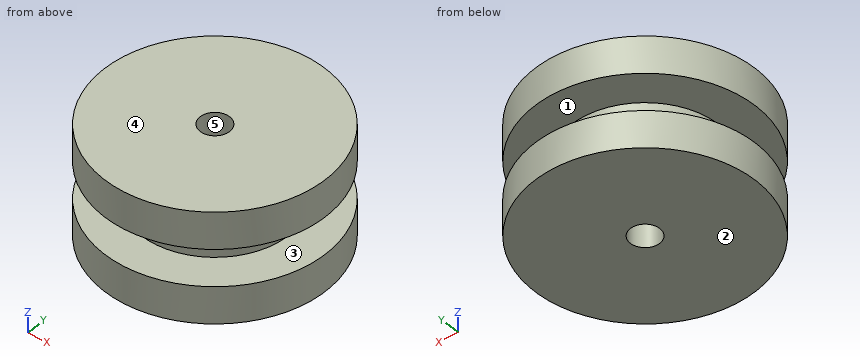
```python
from build123d import *

# Parameters (mm, degrees)
SKETCH1_R          = 20
EXTRUDE1_DEPTH     = 5
SKETCH2_R          = 30
EXTRUDE2_DEPTH     = 10
EXTRUDE3_START     = 10
SKETCH3_R          = 30
EXTRUDE3_DEPTH     = 10
SKETCH4_R          = 4
CUT_EXTRUDE1_DEPTH = 30


with BuildPart() as part:
    # Sketch1 → Extrude1 (new, symmetric)
    with BuildSketch(Plane.XY):
        Circle(SKETCH1_R)
    extrude(amount=EXTRUDE1_DEPTH, both=True)

    # Sketch2 → Extrude2 (add)
    with BuildSketch(Plane.XY.offset(5)):
        Circle(SKETCH2_R)
    extrude(amount=EXTRUDE2_DEPTH)

    # Sketch3 → Extrude3 (add)
    with BuildSketch(Plane(origin=(0, 0, -5), x_dir=(-1, 0, 0), z_dir=(0, 0, -1)).offset(EXTRUDE3_START)):
        with Locations(Location((0, 0, 0), (0, 0, 180))):
            Circle(SKETCH3_R)
    extrude(amount=-EXTRUDE3_DEPTH)

    # Sketch4 → Cut-Extrude1 (cut)
    with BuildSketch(Plane(origin=(0, 0, -15), x_dir=(-1, 0, 0), z_dir=(0, 0, -1))):
        Circle(SKETCH4_R)
    extrude(amount=-CUT_EXTRUDE1_DEPTH, mode=Mode.SUBTRACT)


solid = part.part
```
The listing builds one solid part. Answer for the finished solid, in the listing's coordinates (mm). Face numbers are marked on the shaded views. A direction names the side the tool comes from. Coordinates: 2 decimals unless noted, no trailing zeros. Write each loop counter-clockwise with the first axis right and the second up, starting at its lowest first coordinate (ties: lowest second). Pieces come first, ordered by that corner, then holes. Notation, with made-up numbers: (55.5, 24.5) - (73.5, 24.5) arc R26 cw to (73.5, 62.5) - close; hole circle Ø4 at (64, 45.25). An arc over 180 degrees is marked (long way). Return JSON: item names as keys, results as strings. Group by question number.
Q1. Flat-ended cylindrical pins translate along their axes: pin 1 Ø10 at (x, z) = (17.5, -9.5) entering from +Y; pin 2 Ø12 at (y, z) = (19, -4) entering from -X; pin 3 Ø8 at (x, z) = (-11, -12) entering from +Y. Find the tip coordinate at first contact, or state that the pin passes through.
Q2. The part is cut by section C-C on z = -3.75. Write down the section's boundary in (x, y), and give its area (3 significant figures).
Q3. For a pull along Z with two mould halves and no side action, classify the marked faces 3, 4 and 5 as +Z half, -Z half, draft (parallel to the pull), parting line (faces both ways), or undercut.
Q4. The part is cut by section D-D on x = 16. Write down the section's boundary in (y, z).
Q5. Find the intervals of material crossed by line 1 along Z through (x, y) = (24.5, 13); line 2 along Y through (x, z) = (0, -7.75); line 3 along Y through (x, z) = (0, 0.75), in increasing order. Write a range as [from, to].
Q6. The part is cut by section A-A on x = 0. Write down the section's boundary in (y, z).
Q7. Which of the six approach directions +Z, -Z, +X, -X, +Y, -Y give full straight-line access (tool end or side, diameter ignored) to the marked faces 1 and 2?
Evaluation:
{
 "1": {"pin 1": "stops at y = 27.27", "pin 2": "stops at x = -27", "pin 3": "stops at y = 29.17"},
 "2": {"outline": "circle Ø40 at (0, 0); hole circle Ø8 at (0, 0)", "area": "1,210 mm2"},
 "3": {"face 3": "undercut", "face 4": "+Z half", "face 5": "draft"},
 "4": {"outline": "(-25.38, -15) - (25.38, -15) - (25.38, -5) - (12, -5) - (12, 5) - (25.38, 5) - (25.38, 15) - (-25.38, 15) - (-25.38, 5) - (-12, 5) - (-12, -5) - (-25.38, -5) - close"},
 "5": {"line 1": "z = [-15, -5], [5, 15]", "line 2": "y = [-30, -4], [4, 30]", "line 3": "y = [-20, -4], [4, 20]"},
 "6": {"outline": "(-30, -15) - (-4, -15) - (-4, 15) - (-30, 15) - (-30, 5) - (-20, 5) - (-20, -5) - (-30, -5) - close; (4, -15) - (30, -15) - (30, -5) - (20, -5) - (20, 5) - (30, 5) - (30, 15) - (4, 15) - close"},
 "7": {"face 1": "none", "face 2": "-Z, +X, -X, +Y, -Y"}
}
